```python
from build123d import *

# Parameters (mm, degrees)
SKETCH2_R           = 1.5
BOSS_EXTRUDE1_DEPTH = 27
SKETCH3_R           = 1.5
SKETCH3_W           = 63
SKETCH3_H           = 3.5
BOSS_EXTRUDE2_DEPTH = 2
CHAMFER1_SIZE       = 0.5
CUT_EXTRUDE1_DEPTH  = 11


with BuildPart() as part:
    # Sketch2 → Boss-Extrude1 (new body)
    with BuildSketch(Plane.XY):
        with BuildLine():
            Line((32.824573519, -3.5), (-32.824573519, -3.5))
            Line((-32.824573519, -3.5), (-33.401923789, -4.5))
            Line((-33.401923789, -4.5), (-38.598076211, -4.5))
            Line((-38.598076211, -4.5), (-39.897114317, -2.25))
            ThreePointArc((-39.897114317, -2.25), (-40.5, 0), (-39.897114317, 2.25))
            Line((-39.897114317, 2.25), (-38.598076211, 4.5))
            Line((-38.598076211, 4.5), (-33.401923789, 4.5))
            Line((-33.401923789, 4.5), (-32.824573519, 3.5))
            Line((-32.824573519, 3.5), (32.824573519, 3.5))
            Line((32.824573519, 3.5), (33.401923789, 4.5))
            Line((33.401923789, 4.5), (38.598076211, 4.5))
            Line((38.598076211, 4.5), (39.897114317, 2.25))
            ThreePointArc((39.897114317, 2.25), (40.5, 0), (39.897114317, -2.25))
            Line((39.897114317, -2.25), (38.598076211, -4.5))
            Line((38.598076211, -4.5), (33.401923789, -4.5))
            Line((33.401923789, -4.5), (32.824573519, -3.5))
        make_face()
        with Locations((-36, 0)):
            Circle(SKETCH2_R, mode=Mode.SUBTRACT)
        with Locations((36, 0)):
            Circle(SKETCH2_R, mode=Mode.SUBTRACT)
        Polygon((-27.701125682, 1.75), (-26.427229863, -1.75), (-28.427229863, -1.75), (-29.701125682, 1.75), align=None, mode=Mode.SUBTRACT)
        Polygon((-25.701125682, 1.75), (-24.427229863, -1.75), (-22.427229863, -1.75), (-23.701125682, 1.75), align=None, mode=Mode.SUBTRACT)
        Polygon((-21.701125682, 1.75), (-20.427229863, -1.75), (-18.427229863, -1.75), (-19.701125682, 1.75), align=None, mode=Mode.SUBTRACT)
        Polygon((-17.701125682, 1.75), (-16.427229863, -1.75), (-14.427229863, -1.75), (-15.701125682, 1.75), align=None, mode=Mode.SUBTRACT)
        Polygon((-13.701125682, 1.75), (-12.427229863, -1.75), (-10.427229863, -1.75), (-11.701125682, 1.75), align=None, mode=Mode.SUBTRACT)
        Polygon((-9.701125682, 1.75), (-8.427229863, -1.75), (-6.427229863, -1.75), (-7.701125682, 1.75), align=None, mode=Mode.SUBTRACT)
        Polygon((-5.701125682, 1.75), (-4.427229863, -1.75), (-2.427229863, -1.75), (-3.701125682, 1.75), align=None, mode=Mode.SUBTRACT)
        Polygon((-1.701125682, 1.75), (-0.427229863, -1.75), (1.701125682, -1.75), (0.427229863, 1.75), align=None, mode=Mode.SUBTRACT)
        Polygon((2.427229863, 1.75), (3.701125682, -1.75), (5.701125682, -1.75), (4.427229863, 1.75), align=None, mode=Mode.SUBTRACT)
        Polygon((6.427229863, 1.75), (7.701125682, -1.75), (9.701125682, -1.75), (8.427229863, 1.75), align=None, mode=Mode.SUBTRACT)
        Polygon((10.427229863, 1.75), (11.701125682, -1.75), (13.701125682, -1.75), (12.427229863, 1.75), align=None, mode=Mode.SUBTRACT)
        Polygon((14.427229863, 1.75), (15.701125682, -1.75), (17.701125682, -1.75), (16.427229863, 1.75), align=None, mode=Mode.SUBTRACT)
        Polygon((18.427229863, 1.75), (19.701125682, -1.75), (21.701125682, -1.75), (20.427229863, 1.75), align=None, mode=Mode.SUBTRACT)
        Polygon((22.427229863, 1.75), (23.701125682, -1.75), (25.701125682, -1.75), (24.427229863, 1.75), align=None, mode=Mode.SUBTRACT)
        Polygon((26.427229863, 1.75), (27.701125682, -1.75), (29.701125682, -1.75), (28.427229863, 1.75), align=None, mode=Mode.SUBTRACT)
    extrude(amount=BOSS_EXTRUDE1_DEPTH)

    # Sketch3 → Boss-Extrude2 (add)
    with BuildSketch(Plane.XY.offset(27)):
        with BuildLine():
            Line((-39.897114317, -2.25), (-38.598076211, -4.5))
            Line((-38.598076211, -4.5), (-33.401923789, -4.5))
            Line((-33.401923789, -4.5), (-32.824573519, -3.5))
            Line((-32.824573519, -3.5), (32.824573519, -3.5))
            Line((32.824573519, -3.5), (33.401923789, -4.5))
            Line((33.401923789, -4.5), (38.598076211, -4.5))
            Line((38.598076211, -4.5), (39.897114317, -2.25))
            ThreePointArc((39.897114317, -2.25), (40.5, 0), (39.897114317, 2.25))
            Line((39.897114317, 2.25), (38.598076211, 4.5))
            Line((38.598076211, 4.5), (33.401923789, 4.5))
            Line((33.401923789, 4.5), (32.824573519, 3.5))
            Line((32.824573519, 3.5), (-32.824573519, 3.5))
            Line((-32.824573519, 3.5), (-33.401923789, 4.5))
            Line((-33.401923789, 4.5), (-38.598076211, 4.5))
            Line((-38.598076211, 4.5), (-39.897114317, 2.25))
            ThreePointArc((-39.897114317, 2.25), (-40.5, 0), (-39.897114317, -2.25))
        make_face()
        with Locations((-36, 0)):
            Circle(SKETCH3_R, mode=Mode.SUBTRACT)
        with Locations((36, 0)):
            Circle(SKETCH3_R, mode=Mode.SUBTRACT)
        Rectangle(SKETCH3_W, SKETCH3_H, mode=Mode.SUBTRACT)
    extrude(amount=BOSS_EXTRUDE2_DEPTH)

    # Chamfer1
    chamfer1_edges = [part.edges().sort_by_distance(p)[0] for p in [
        (-9.064177772, 0, 27),
        (-7.064177772, 0, 27),
        (-5.064177772, 0, 27),
        (-3.064177772, 0, 27),
        (-1.064177772, 0, 27),
        (1.064177772, 0, 27),
        (3.064177772, 0, 27),
        (5.064177772, 0, 27),
        (7.064177772, 0, 27),
        (9.064177772, 0, 27),
        (11.064177772, 0, 27),
        (13.064177772, 0, 27),
        (15.064177772, 0, 27),
        (17.064177772, 0, 27),
        (19.064177772, 0, 27),
        (21.064177772, 0, 27),
        (23.064177772, 0, 27),
        (25.064177772, 0, 27),
        (27.064177772, 0, 27),
        (29.064177772, 0, 27),
        (0, -3.5, 29),
        (0, 3.5, 29),
        (0, 1.75, 29),
        (0, -1.75, 29),
        (-29.064177772, 0, 27),
        (-27.064177772, 0, 27),
        (-25.064177772, 0, 27),
        (-23.064177772, 0, 27),
        (-21.064177772, 0, 27),
        (-19.064177772, 0, 27),
        (-17.064177772, 0, 27),
        (-15.064177772, 0, 27),
        (-13.064177772, 0, 27),
        (-11.064177772, 0, 27),
    ]]
    chamfer(chamfer1_edges, length=CHAMFER1_SIZE)

    # Sketch4 → Cut-Extrude1 (cut, symmetric)
    with BuildSketch(Plane.XY.offset(14.5)):
        with BuildLine():
            Line((-33.401923789, 4.5), (-34.844518305, 6.998646998))
            Line((-34.844518305, 6.998646998), (10.516878585, 6.998646998))
            Line((10.516878585, 6.998646998), (12.427229863, 1.75))
            Line((12.427229863, 1.75), (13.701125682, -1.75))
            Line((13.701125682, -1.75), (15.61147696, -6.998646998))
            Line((15.61147696, -6.998646998), (-34.844518305, -6.998646998))
            Line((-34.844518305, -6.998646998), (-33.401923789, -4.5))
            Line((-33.401923789, -4.5), (-32.102885683, -2.25))
            ThreePointArc((-32.102885683, -2.25), (-31.5, 0), (-32.102885683, 2.25))
            Line((-32.102885683, 2.25), (-33.401923789, 4.5))
        make_face()
    extrude(amount=CUT_EXTRUDE1_DEPTH, both=True, mode=Mode.SUBTRACT)


solid = part.part
```
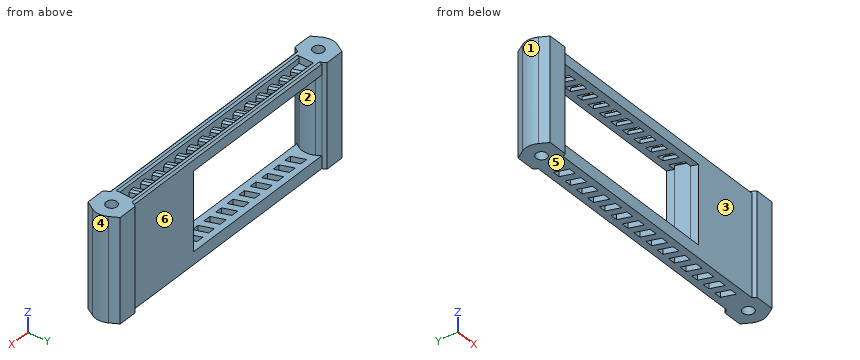
Design review of the part built by this model. Coordinates are the model's own, in mm. Face numbers are marked on the shaded views. A direction names the side the tool comes from. Give positions to 0.01 mm unless a question says otherwise; leave off trailing zeros. Loops run counter-clockwise (first coordinate to the right, second up) from the corner with the lowest first, then second, coordinate; pieces in that order, holes last. Notation, with made-up numbers: (-34.75, 79) -> (14.25, 79) arc R36 cw to (14.25, 118) -> close; hole circle Ø3 at (39.25, -16). An arc over 180 degrees is marked (long way). Write each question's results on one line, items separated by ' | '.
Q1. Machinability: for the marked faces 5 and 6, which of the approach directions +Z, -Z, +X, -X, +Y, -Y give a long, thin tool a straight path to every point of the face, cutting with its end or side? Answer none if there is none.
Reply:
face 5: -Z, +X, -X, +Y, -Y | face 6: +Z, -Z, +Y
Q2. Wall thickness on L1, parallel to Y at x = -36, z = 11.25; L2, parallel to Z at x = -20, y = 2.5; L3, parallel to X at y = -2.25, z = 17: over which ranges is each line inside the solid? List them lowest first.
Reply:
L1: y = -4.5 to -1.5, 1.5 to 4.5 | L2: z = 0 to 3.5, 25.5 to 29 | L3: x = -39.9 to -32.1, 13.88 to 39.9
Q3. Take a section at B-B, the plane z = 11.5. Give the number of separate pieces and of enclosed holes in the cut face, plus the area to 3 significant figures.
Reply:
separate pieces: 2 | enclosed holes: 6 | area: 226 mm²
Q4. Take a section at A-A, the plane x = -36. Write out the cut boundary in (y, z).
Reply:
outline: (-4.5, 0) -> (-1.5, 0) -> (-1.5, 29) -> (-4.5, 29) -> close; (1.5, 0) -> (4.5, 0) -> (4.5, 29) -> (1.5, 29) -> close
Q5. For pin 1 Ø1 at (x, z) = (-13, 1) entering from -Y; pin 2 Ø2.5 at (x, y) = (-18.5, 0) entering from +Z; pin 3 Ø1.6 at (x, z) = (12.5, 2) entering from +Y; pin 4 Ø2.5 at (x, y) = (-36, 0) entering from +Z, all flat-tipped, find the tip position at first contact; note any pin that passes through.
Reply:
pin 1: stops at y = -3.5 | pin 2: stops at z = 27 | pin 3: stops at y = 3.5 | pin 4: passes through
Q6. The part is to be moulded in two halves that separate along X. For the marked faces 1, 2, 3 and 4, say which applies: +X half, -X half, draft (parallel to the pull), parting line (faces both ways), or undercut.
Reply:
face 1: -X half | face 2: undercut | face 3: undercut | face 4: +X half
